Build history of the part. All positions in model axes, mm. Give positions to 0.01 mm unless a question says otherwise; leave off trailing zeros. Loops run counter-clockwise (first coordinate to the right, second up) from the corner with the lowest first, then second, coordinate; pieces in that order, holes last.
1) Band-saw the part on A-A on x = -8.5. List the corners of the cut face in (y, z), then the cut area to 3 significant figures.
2) Band-saw the part on D-D on z = 5. State how many separate pieces and enclosed holes the cut face has, then the cut area to 3 significant figures.
3) Band-saw the part on B-B on y = 36. List the corners of the cut face in (x, z).
4) Flat gauge pins, fed straight in: P1, Ø1, axis at x = -11, y = 44, coming from the +Z side; P2, Ø2.5, axis at x = 78.5, y = -58, coming from the +Z side; P3, Ø3, axis at y = -67.5, z = 3.5, coming from the -X side. Where does each tip first touch, or does it go through?
5) Band-saw the part on C-C on x = 89.5. List the corners of the cut face in (y, z).
6) Wall check: line 1 (Y direction, x = -48.5, z = 6.5); line 2 (Z direction, x = 105, y = -67); line 3 (X direction, y = -13.5, z = 6). Give the ranges that are in metal, low to high.
```python
from build123d import *

# Parameters (mm, degrees)
CROQUIS1_W              = 218
CROQUIS1_H              = 145
SALIENTE_EXTRUIR1_DEPTH = 10
CORTAR_EXTRUIR1_DEPTH   = 7
CROQUIS3_W              = 157.5
CROQUIS3_H              = 90
CORTAR_EXTRUIR2_DEPTH   = 4
CHAFL_N1_SIZE           = 2
CORTAR_EXTRUIR3_START   = -2
CROQUIS4_R              = 1.95
CORTAR_EXTRUIR3_DEPTH   = 9
CROQUIS5_W              = 22
CROQUIS5_H              = 55
CROQUIS5_W_2            = 16
CROQUIS5_H_2            = 76.408682756
CROQUIS5_W_3            = 50
CROQUIS5_H_3            = 16
CORTAR_EXTRUIR4_DEPTH   = 7
CROQUIS8_R              = 2.1
CORTAR_EXTRUIR6_DEPTH   = 219
CROQUIS9_R              = 3.5
CORTAR_EXTRUIR7_DEPTH   = 6
CHAFL_N2_SIZE           = 3
CROQUIS10_W             = 30
CROQUIS10_H             = 10.660254038
CORTAR_EXTRUIR8_DEPTH   = 11
CHAFL_N3_SIZE           = 1


with BuildPart() as part:
    # Croquis1 → Saliente-Extruir1 (new body)
    with BuildSketch(Plane.XY):
        Rectangle(CROQUIS1_W, CROQUIS1_H)
    extrude(amount=SALIENTE_EXTRUIR1_DEPTH)

    # Croquis2 → Cortar-Extruir1 (cut)
    with BuildSketch(Plane.XY.offset(10)):
        Polygon((-83, 43), (-83, 48), (82.7, 48), (82.7, -53), (80.5, -53), (-83, -53), align=None)
    extrude(amount=-CORTAR_EXTRUIR1_DEPTH, mode=Mode.SUBTRACT)

    # Croquis3 → Cortar-Extruir2 (cut, through all)
    with BuildSketch(Plane.XY.offset(3)):
        with Locations((-1.25, -5)):
            Rectangle(CROQUIS3_W, CROQUIS3_H)
    extrude(amount=-CORTAR_EXTRUIR2_DEPTH, mode=Mode.SUBTRACT)

    # Chaflán1
    chafl_n1_edges = [part.edges().sort_by_distance(p)[0] for p in [
        (-80, -5, 0),
        (-1.25, 40, 0),
        (77.5, -5, 0),
        (-1.25, -50, 0),
    ]]
    chamfer(chafl_n1_edges, length=CHAFL_N1_SIZE)

    # Croquis4 → Cortar-Extruir3 (cut, through all)
    with BuildSketch(Plane(origin=(0, 0, 0), x_dir=(-1, 0, 0), z_dir=(0, 0, -1)).offset(CORTAR_EXTRUIR3_START)):
        with Locations((-78.5, 56.5)):
            Circle(CROQUIS4_R)
        with Locations((78.5, 56.5)):
            Circle(CROQUIS4_R)
        with Locations((78.5, -58)):
            Circle(CROQUIS4_R)
        with Locations((-78.5, -58)):
            Circle(CROQUIS4_R)
    extrude(amount=-CORTAR_EXTRUIR3_DEPTH, mode=Mode.SUBTRACT)

    # Croquis5 → Cortar-Extruir4 (cut)
    with BuildSketch(Plane.XY.offset(10)):
        with Locations((93.7, -25.5)):
            Rectangle(CROQUIS5_W, CROQUIS5_H)
        with Locations((-91, 0)):
            Rectangle(CROQUIS5_W_2, CROQUIS5_H_2)
        with Locations((0, 56)):
            Rectangle(CROQUIS5_W_3, CROQUIS5_H_3)
        with Locations((0, -56)):
            Rectangle(CROQUIS5_W_3, CROQUIS5_H_3)
    extrude(amount=-CORTAR_EXTRUIR4_DEPTH, mode=Mode.SUBTRACT)

    # Croquis8 → Cortar-Extruir6 (cut, through all)
    with BuildSketch(Plane.ZY.offset(109)):
        with Locations((5, -67.5)):
            Circle(CROQUIS8_R)
    extrude(amount=-CORTAR_EXTRUIR6_DEPTH, mode=Mode.SUBTRACT)

    # Croquis9 → Cortar-Extruir7 (cut)
    with BuildSketch(Plane.ZY.offset(109)):
        with Locations((5, -67.5)):
            Circle(CROQUIS9_R)
    cortar_extruir7 = extrude(amount=-CORTAR_EXTRUIR7_DEPTH, mode=Mode.SUBTRACT)

    # Simetría1: Cortar-Extruir7 across plane
    add(cortar_extruir7.mirror(Plane(origin=(0, 0, 0), x_dir=(0, 0, 1), z_dir=(1, 0, 0))), mode=Mode.SUBTRACT)

    # Chaflán2
    chafl_n2_edges = [part.edges().sort_by_distance(p)[0] for p in [
        (0, 72.5, 10),
        (0, 72.5, 0),
        (0, -72.5, 0),
        (0, -72.5, 10),
    ]]
    chamfer(chafl_n2_edges, length=CHAFL_N2_SIZE)

    # Croquis10 → Cortar-Extruir8 (cut, through all)
    with BuildSketch(Plane(origin=(0, 0, 0), x_dir=(-1, 0, 0), z_dir=(0, 0, -1))):
        with Locations((-50, -67.169872981)):
            Rectangle(CROQUIS10_W, CROQUIS10_H)
        with Locations((50, -67.169872981)):
            Rectangle(CROQUIS10_W, CROQUIS10_H)
    extrude(amount=-CORTAR_EXTRUIR8_DEPTH, mode=Mode.SUBTRACT)

    # Chaflán3
    chafl_n3_edges = [part.edges().sort_by_distance(p)[0] for p in [
        (80.45, -58, 10),
        (-76.55, -58, 10),
        (-76.55, 56.5, 10),
        (80.45, 56.5, 10),
    ]]
    chamfer(chafl_n3_edges, length=CHAFL_N3_SIZE)


solid = part.part
```
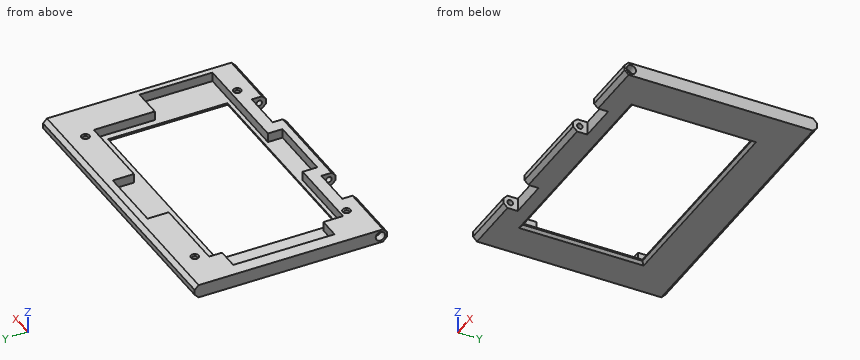
Findings below:
1. outline: (-72.5, 3) - (-69.5, 0) - (-52, 0) - (-50, 2) - (-50, 3) - (-64, 3) - (-64, 10) - (-69.5, 10) - (-72.5, 7) - close; (40, 2) - (42, 0) - (69.5, 0) - (72.5, 3) - (72.5, 7) - (69.5, 10) - (64, 10) - (64, 3) - (40, 3) - close; hole circle Ø4.2 at (-67.5, 5)
1. area: 248 mm2
2. separate pieces: 4
2. enclosed holes: 5
2. area: 9,710 mm2
3. outline: (-109, 0) - (-82, 0) - (-80, 2) - (-80, 3) - (-99, 3) - (-99, 10) - (-109, 10) - close; (77.5, 2) - (79.5, 0) - (109, 0) - (109, 10) - (82.7, 10) - (82.7, 3) - (77.5, 3) - close
4. P1: stops at z = 3
4. P2: stops at z = 2
4. P3: stops at x = -103
5. outline: (-72.5, 3) - (-69.5, 0) - (69.5, 0) - (72.5, 3) - (72.5, 7) - (69.5, 10) - (2, 10) - (2, 3) - (-53, 3) - (-53, 10) - (-69.5, 10) - (-72.5, 7) - close; hole circle Ø4.2 at (-67.5, 5)
6. line 1: y = -61.84 to -53, 48 to 72.5
6. line 2: z = 0 to 1.54, 8.46 to 10
6. line 3: x = -109 to -99, 104.7 to 109
